from build123d import *

# Parameters (mm, degrees)
SKETCH3_W             = 300
SKETCH3_H             = 500
BOSS_EXTRUDE2_DEPTH   = 50
BOSS_EXTRUDE3_DEPTH   = 50
BOSS_EXTRUDE4_DEPTH   = 50
SKETCH7_R             = 15
BOSS_EXTRUDE5_DEPTH   = 200
BOSS_EXTRUDE6_DEPTH   = 15
SKETCH9_W             = 20
SKETCH9_H             = 20
BOSS_EXTRUDE7_DEPTH   = 100
SKETCH10_W            = 75
SKETCH10_H            = 75
BOSS_EXTRUDE8_DEPTH   = 20
BODY_MOVE_COPY1_ANGLE = 89


with BuildPart() as part:
    # Sketch3 → Boss-Extrude2 (new body)
    with BuildSketch(Plane.XY):
        Rectangle(SKETCH3_W, SKETCH3_H)
    extrude(amount=BOSS_EXTRUDE2_DEPTH)

    # Sketch5 → Boss-Extrude3 (add)
    with BuildSketch(Plane.ZY.offset(150)):
        Polygon((50, 250), (125, 200), (125, 100), (50, 50), align=None)
        Polygon((50, -50), (50, -250), (125, -200), (125, -100), align=None)
    extrude(amount=-BOSS_EXTRUDE3_DEPTH)

    # Sketch6 → Boss-Extrude4 (add)
    with BuildSketch(Plane(origin=(150, 0, 0), x_dir=(0, 0, -1), z_dir=(1, 0, 0))):
        Polygon((-50, -250), (-50, -50), (-125, -100), (-125, -200), align=None)
        Polygon((-50, 250), (-125, 200), (-125, 100), (-50, 50), align=None)
    extrude(amount=-BOSS_EXTRUDE4_DEPTH)

    # Sketch7 → Boss-Extrude5 (add)
    with BuildSketch(Plane.XY.offset(50)):
        with Locations((-100, 150)):
            Circle(SKETCH7_R)
        with Locations((100, 150)):
            Circle(SKETCH7_R)
        with Locations((-100, -150)):
            Circle(SKETCH7_R)
        with Locations((100, -150)):
            Circle(SKETCH7_R)
    extrude(amount=BOSS_EXTRUDE5_DEPTH)

    # Sketch8 → Boss-Extrude6 (add)
    with BuildSketch(Plane.XY.offset(250)):
        with BuildLine():
            Line((-115, 150.000000362), (-115, -150))
            ThreePointArc((-115, -150), (-110.606601718, -160.606601718), (-100, -165))
            Line((-100, -165), (100.000000138, -165))
            ThreePointArc((100.000000138, -165), (110.606601767, -160.606601669), (115, -150))
            Line((115, -150), (115, 150))
            ThreePointArc((115, 150), (110.606601718, 160.606601718), (100, 165))
            Line((100, 165), (-100, 165))
            ThreePointArc((-100, 165), (-110.60660159, 160.606601846), (-115, 150.000000362))
        make_face()
    extrude(amount=BOSS_EXTRUDE6_DEPTH)

    # Sketch9 → Boss-Extrude7 (add)
    with BuildSketch(Plane.XY.offset(50)):
        with Locations((0, 240)):
            Rectangle(SKETCH9_W, SKETCH9_H)
    extrude(amount=BOSS_EXTRUDE7_DEPTH)

    # Sketch10 → Boss-Extrude8 (add)
    with BuildSketch(Plane(origin=(0, 250, 0), x_dir=(1, 0, 0), z_dir=(0, 1, 0))):
        with Locations((0, -150)):
            Rectangle(SKETCH10_W, SKETCH10_H)
    extrude(amount=-BOSS_EXTRUDE8_DEPTH)


with BuildPart() as part_1:
    # Body-Move/Copy1: moved
    add(part.part.rotate(Axis((0, 0, 0), (0, 0, -1)), BODY_MOVE_COPY1_ANGLE))


solid = part_1.part
Here's how the part is built. I have some questions about the finished solid (model axes, mm). A direction names the side the tool comes from. Coordinates: 2 decimals unless noted, no trailing zeros. Order: outer loops, then holes, each group sorted by start corner. A loop starts at its lowest first (then second) coordinate and runs counter-clockwise, first axis right, second up.
Item 1: I need wall thicknesses on line 1 (Z direction, x = -107, y = -33.5); line 2 (Z direction, x = 124.5, y = 113); line 3 (Y direction, x = -146.5, z = 159). Which ranges of each line are inside material? Lowest first, please.
Result sheet:
line 1: z = 0 to 50, 250 to 265
line 2: z = 0 to 125, 250 to 265
line 3: y = -117.5 to -87.7, 83.31 to 111.43
Item 2: If we section it at B-B on z = 91: List the corners of the cut face in (x, y) for me.
Result sheet:
outline: (-225.25, 146.09) - (-224.38, 96.1) - (-166.72, 97.11) arc R15 ccw to (-136.72, 97.63) - (-79.07, 98.64) - (-79.94, 148.63) - close; (-220.89, -103.87) - (-220.01, -153.86) - (-74.7, -151.33) - (-75.58, -101.33) - (-133.23, -102.34) arc R15 ccw to (-163.23, -102.86) - close; (74.7, 151.33) - (75.58, 101.33) - (133.23, 102.34) arc R15 ccw to (163.23, 102.86) - (220.89, 103.87) - (220.01, 153.86) - close; (79.07, -98.64) - (79.94, -148.63) - (225.25, -146.09) - (224.38, -96.1) - (166.72, -97.11) arc R15 ccw to (136.72, -97.63) - close; (229.79, 14.01) - (230.14, -5.98) - (250.14, -5.64) - (249.79, 14.36) - close
Item 3: If we section it at C-C on y = 65: List the corners of the cut face in (x, z) for me, plus the area to 3 significant figures.
Result sheet:
outline: (-251.17, 0) - (248.9, 0) - (248.9, 50) - (-251.17, 50) - close; (-166.16, 250) - (163.89, 250) - (163.89, 265) - (-166.16, 265) - close
area: 30,000 mm2
Item 4: For faces 1 (the face through (2, 2, 250)), 2 (the face through (3, 2, 0)), 3 (the face through (-147, -128, 125)), which set-ups out of +Z, -Z, +X, -X, +Y, -Y let a thin tool reach every point of the face, with its end or its side?
Result sheet:
face 1: none
face 2: -Z, +X, -X, +Y, -Y
face 3: -Y
Item 5: If we section it at D-D on y = -128.5: List the corners of the cut face in (x, z) for me, plus the area to 3 significant figures.
Result sheet:
outline: (-247.8, 0) - (252.28, 0) - (252.28, 50) - (202.27, 125) - (102.26, 125) - (52.25, 50) - (-47.76, 50) - (-97.77, 125) - (-197.79, 125) - (-247.8, 50) - close
area: 47,500 mm2
Item 6: For P1, Ø12, axis at x = 182, z = 36, coming from the +Y side; P2, Ø2, axis at x = -79, z = 89, coming from the +Y side; P3, Ø8, axis at y = 101.5, z = 74.5, coming from the -X side; P4, Ø16.5, axis at x = 244.5, y = -25, coming from the -Z side, each with a flat end and sliding along its axis, tell me the tip position at first contact or that it passes through.
Result sheet:
P1: stops at y = 153.3
P2: stops at y = 148.66
P3: stops at x = -238.14
P4: stops at z = 0
Item 7: If we section it at A-A on x = -109: List the corners of the cut face in (y, z) for me, plus the area to 3 significant figures.
Result sheet:
outline: (-151.93, 0) - (148.12, 0) - (148.12, 125) - (98.11, 125) - (98.11, 50) - (-101.92, 50) - (-101.92, 125) - (-151.93, 125) - close; (-116.92, 250) - (113.11, 250) - (113.11, 265) - (-116.92, 265) - close
area: 26,000 mm2
